Work out the finished part from the listing and answer in its coordinate system (mm). A direction names the side the tool comes from. Give positions to 0.01 mm unless a question says otherwise; leave off trailing zeros. Loops run counter-clockwise (first coordinate to the right, second up) from the corner with the lowest first, then second, coordinate; pieces in that order, holes last.
from build123d import *

# Parameters (mm, degrees)
F0_R     = 12.7
F1_DEPTH = 25.4
F2_R     = 6.35
F5_DEPTH = 19.05
F6_W     = 7.035027858
F6_H     = 7.62
F7_DEPTH = 25.4
F8_DEPTH = 2.54


with BuildPart() as f1:
    # F0 (on Top) → F1 (new body)
    with BuildSketch(Plane.XY):
        Circle(F0_R)
    extrude(amount=F1_DEPTH)

    # F2 (on face) + F4 (on face) + F3 (on face) → F5 (cut)
    with BuildSketch(Plane.XY.offset(25.4)):
        Circle(F2_R)
    with BuildSketch(Plane.XY.offset(25.4)):
        with BuildLine():
            Line((0, 12.7), (0, 6.35))
            ThreePointArc((0, 6.35), (2.0080463142, 6.0241389426), (3.81, 5.08))
            Line((3.81, 5.08), (3.81, 12.7))
            Line((3.81, 12.7), (0, 12.7))
        make_face()
    with BuildSketch(Plane.XY.offset(25.4)):
        with BuildLine():
            ThreePointArc((-3.81, 5.08), (-2.0080463142, 6.0241389426), (0, 6.35))
            Line((0, 6.35), (0, 12.7))
            Line((0, 12.7), (-3.81, 12.7))
            Line((-3.81, 12.7), (-3.81, 5.08))
        make_face()
    extrude(amount=-F5_DEPTH, mode=Mode.SUBTRACT)

    # F6 (on face) → F7 (cut)
    with BuildSketch(Plane(origin=(3.81, 0, 0), x_dir=(0, -1, 0), z_dir=(-1, 0, 0))):
        with Locations((-8.597513929, 10.16)):
            Rectangle(F6_W, F6_H)
    extrude(amount=-F7_DEPTH, mode=Mode.SUBTRACT)

    # F8 (cut): a face of the model
    f8_faces = [f1.faces().sort_by_distance(p)[0] for p in [
        (7.7248711326, 5.08, 10.16),
    ]]
    extrude(f8_faces, amount=-F8_DEPTH, mode=Mode.SUBTRACT)


solid = f1.part
Item 1: Find section C-C, the plane z = 10.5. Write down the section's boundary in (x, y).
Item 2: For faces 5 (the face through (-0.222, -6.346, 16.008)), 6 (the face through (-3.81, 9, 16)), 7 (the face through (0, 0, 0)), 8 (the face through (9, 2.54, 10)), determine the directions among +Z, -Z, +X, -X, +Y, -Y from which every point of the face is accessible in a straight line to the end or side of a thin tool.
Item 3: Determine the mould class of faces 1 (the face through (11.64, 4, 10)), 2 (the face through (1, 3, 6.35)), 3 (the face through (-2.75, -12.4, 12.52)), 4 (the face through (-3, -6, 25.4)) for opening direction X: released by +X, released by -X, zero draft, split by the parting line, or undercut.
Item 4: Flat-ended cylindrical pins translate along their axes: pin 1 Ø1 at (x, z) = (-1, 20) entering from +Y; pin 2 Ø4 at (y, z) = (-8, 5) entering from -X; pin 3 Ø7.5 at (y, z) = (9, 19) entering from -X. Find the tip coordinate at first contact, or state that the pin passes through.
Item 5: Find section A-A, the plane x = 0. Write down the section's boundary in (y, z).
Item 6: Find section D-D, the plane y = 0. Write down the section's boundary in (x, z), plus the area to 3 significant figures.
Item 7: Consider line 1 (X direction, y = 0, z = 19.25); line 2 (X direction, y = 11, z = 19); line 3 (Z direction, x = 6, y = -1). Determine where each line is inside the solid, lowest interval first.
Item 8: Find section B-B, the plane y = 10. Write down the section's boundary in (x, z), plus the area to 3 significant figures.
Ans:
1. outline: (-3.81, 5.08) - (-3.81, 12.12) arc R12.7 ccw (long way) to (11.64, 5.08) - (11.64, 2.54) - (5.82, 2.54) arc R6.35 cw (long way) to start
2. face 5: +Z
2. face 6: +Z, +Y
2. face 7: -Z, +X, -X, +Y, -Y
2. face 8: +Y
3. face 1: undercut
3. face 2: undercut
3. face 3: split by the parting line
3. face 4: zero draft
4. pin 1: stops at y = -6.17
4. pin 2: stops at x = -11.19
4. pin 3: stops at x = -11.56
5. outline: (-12.7, 0) - (12.7, 0) - (12.7, 6.35) - (-6.35, 6.35) - (-6.35, 25.4) - (-12.7, 25.4) - close
6. outline: (-12.7, 0) - (12.7, 0) - (12.7, 25.4) - (6.35, 25.4) - (6.35, 6.35) - (-6.35, 6.35) - (-6.35, 25.4) - (-12.7, 25.4) - close
6. area: 403 mm2
7. line 1: x = -12.7 to -6.35, 6.35 to 12.7
7. line 2: x = -6.35 to -3.81, 3.81 to 6.35
7. line 3: z = 0 to 6.35
8. outline: (-7.83, 0) - (7.83, 0) - (7.83, 6.35) - (-3.81, 6.35) - (-3.81, 25.4) - (-7.83, 25.4) - close; (3.81, 13.97) - (7.83, 13.97) - (7.83, 25.4) - (3.81, 25.4) - close
8. area: 222 mm2
